```python
from build123d import *

# Parameters (mm, degrees)
MAIN_BLOCK_DEPTH                = 15
TENSION_SCREW_HOLES_D           = 3.4
TENSION_SCREW_HOLES_CBORE_D     = 6.5
TENSION_SCREW_HOLES_CBORE_DEPTH = 3.4
IDLER_MOUNTING_HOLE_D           = 5
COSMETIC_CHAMFER_SIZE           = 2
PRINT_HELPER_FILLETS_R          = 2
COSMETIC_CHAMFERS_SIZE          = 2


with BuildPart() as part:
    # Main Body Sketch → Main Block (new body)
    with BuildSketch(Plane(origin=(0, 0, 0), x_dir=(1, 0, 0), z_dir=(0, 1, 0))):
        Polygon((-12.5, 20), (-12.5, 10), (-25, 10), (-25, 0), (-25, -5), (25, -5), (25, 10), (12.5, 10), (12.5, 20), (5.5, 20), (5.5, 5), (-5.5, 5), (-5.5, 20), align=None)
    extrude(amount=MAIN_BLOCK_DEPTH)

    # Tension Screw Holes (through all)
    with Locations(Plane(origin=(0, 0, -10), x_dir=(-1, 0, 0), z_dir=(0, 0, -1))):
        with Locations((17.5, 7.5), (-17.5, 7.5)):
            CounterBoreHole(TENSION_SCREW_HOLES_D / 2, TENSION_SCREW_HOLES_CBORE_D / 2, TENSION_SCREW_HOLES_CBORE_DEPTH)

    # Idler Mounting Hole (through all)
    with Locations(Plane(origin=(12.5, 0, 0), x_dir=(0, 0, -1), z_dir=(1, 0, 0))):
        with Locations((15, 7.5)):
            Hole(IDLER_MOUNTING_HOLE_D / 2)

    # Cosmetic Chamfer
    cosmetic_chamfer_edges = [part.edges().sort_by_distance(p)[0] for p in [
        (9, 0, -20),
        (-9, 0, -20),
        (9, 15, -20),
        (-9, 15, -20),
    ]]
    chamfer(cosmetic_chamfer_edges, length=COSMETIC_CHAMFER_SIZE)

    # Print Helper Fillets
    print_helper_fillets_edges = [part.edges().sort_by_distance(p)[0] for p in [
        (-5.5, 7.5, -5),
        (5.5, 7.5, -5),
        (-12.5, 7.5, -20),
        (-5.5, 7.5, -20),
        (5.5, 7.5, -20),
        (12.5, 7.5, -20),
        (-25, 7.5, 5),
        (25, 7.5, -10),
        (25, 7.5, 5),
        (-25, 7.5, -10),
    ]]
    fillet(print_helper_fillets_edges, radius=PRINT_HELPER_FILLETS_R)

    # Cosmetic Chamfers
    cosmetic_chamfers_edges = [part.edges().sort_by_distance(p)[0] for p in [
        (-17.75, 0, -10),
        (-24.414213562, 0, -9.414213562),
        (-25, 0, -2.5),
        (-24.414213562, 0, 4.414213562),
        (0, 0, 5),
        (17.75, 0, -10),
        (24.414213562, 0, 4.414213562),
        (24.414213562, 0, -9.414213562),
        (25, 0, -2.5),
        (-12.5, 0, -14),
        (12.5, 0, -14),
    ]]
    chamfer(cosmetic_chamfers_edges, length=COSMETIC_CHAMFERS_SIZE - 0.0001)  # a hair under: the kernel refuses the full size


solid = part.part
```
Geometry check sheet. Reference: the model listing, model coordinates, mm. A direction names the side the tool comes from. Give positions to 0.01 mm unless a question says otherwise; leave off trailing zeros. Order: outer loops, then holes, each group sorted by start corner. A loop starts at its lowest first (then second) coordinate and runs counter-clockwise, first axis right, second up. Notation, with made-up numbers: (83, 87) -> (126, 87) arc R15 cw to (126, 104) -> close; hole circle Ø8 at (78.5, 70.5). An arc over 180 degrees is marked (long way). Write each question's results on one line, items separated by ' | '. Start each with the question number.
(1) Scan lines: line 1 (Y direction, x = -17.5, z = -7.3); line 2 (Y direction, x = -17.5, z = -1.75); line 3 (X direction, y = 7.75, z = -3.75). Record each from-to range of solid material in increasing order.
(2) Sectioned sample at A-A (x = 9.5). Enter the section's corners in (y, z), plus the area to 3 significant figures.
(3) Sectioned sample at D-D (y = 12). Enter the section's corners in (x, z), plus the area to 3 significant figures.
(4) Gauge pin test, flat ends, axial feed: P1, Ø6, axis at x = 17.5, y = 7.5, coming from the -Z side; P2, Ø3, axis at x = 19, y = 8.5, coming from the -Z side; P3, Ø2.5, axis at x = 17.5, y = 7.5, coming from the -Z side; P4, Ø8, axis at y = 7.5, z = -15, coming from the +X side. Record the tip position at first contact, or that the pin passes through.
(5) Sectioned sample at B-B (z = 2.5). Enter the section's corners in (x, y), plus the area to 3 significant figures.
(6) Mould release check, pull along X, two halves, no side actions. Record for faces 1 (the face through (-11.5, 1, -13.8)), 2 (the face through (-14.253, 7.643, -8.324)), 3 (the face through (11.5, 1, -13.6)): pulls with the +X half, pulls with the -X half, needs draft (parallel to the pull), parting line crosses it, or undercut.
(7) Access from +Z, -Z, +X, -X, +Y, -Y to the whole of each face (thin tool, end or side, straight path). Record for faces 4 (the face through (-23.72, 1.01, 3.71)), 5 (the face through (12.5, 10, -14)), 6 (the face through (-4.93, 7.6, -5.6)), 7 (the face through (-17, 1, -9)).
(8) Sectioned sample at C-C (z = -15). Enter the section's corners in (x, y), plus the area to 3 significant figures.
Answer below:
1) line 1: 0 to 4.25, 10.75 to 15 | line 2: 0 to 5.8, 9.2 to 15 | line 3: -25 to -19.18, -15.82 to 15.82, 19.18 to 25
2) outline: (0, -18) -> (2, -20) -> (13, -20) -> (15, -18) -> (15, 5) -> (2, 5) -> (0, 3) -> close; hole circle Ø5 at (7.5, -15) | area: 349 mm2
3) outline: (-25, -8) arc R2 ccw to (-23, -10) -> (-12.5, -10) -> (-12.5, -18) arc R2 ccw to (-10.5, -20) -> (-7.5, -20) arc R2 ccw to (-5.5, -18) -> (-5.5, -7) arc R2 cw to (-3.5, -5) -> (3.5, -5) arc R2 cw to (5.5, -7) -> (5.5, -18) arc R2 ccw to (7.5, -20) -> (10.5, -20) arc R2 ccw to (12.5, -18) -> (12.5, -10) -> (23, -10) arc R2 ccw to (25, -8) -> (25, 3) arc R2 ccw to (23, 5) -> (-23, 5) arc R2 ccw to (-25, 3) -> close | area: 830 mm2
4) P1: z = -6.6 | P2: z = -10 | P3: through | P4: x = 12.5
5) outline: (-25, 2) -> (-23, 0) -> (23, 0) -> (25, 2) -> (25, 15) -> (-25, 15) -> close; hole circle Ø3.4 at (-17.5, 7.5); hole circle Ø3.4 at (17.5, 7.5) | area: 728 mm2
6) face 1: pulls with the -X half | face 2: undercut | face 3: pulls with the +X half
7) face 4: +Z, -X, -Y | face 5: -Z, +X, +Y, -Y | face 6: -Z, +Y, -Y | face 7: -Z, -X, -Y
8) outline: (-12.5, 2) -> (-10.5, 0) -> (-5.5, 0) -> (-5.5, 5) -> (-12.5, 5) -> close; (-12.5, 10) -> (-5.5, 10) -> (-5.5, 15) -> (-12.5, 15) -> close; (5.5, 0) -> (10.5, 0) -> (12.5, 2) -> (12.5, 5) -> (5.5, 5) -> close; (5.5, 10) -> (12.5, 10) -> (12.5, 15) -> (5.5, 15) -> close | area: 136 mm2
